Here's the drawing with two shaded views (mm, measured from the low corner). I have some questions. Coordinates: 2 decimals unless noted, no trailing zeros. Loops run counter-clockwise (first coordinate to the right, second up) from the corner with the lowest first, then second, coordinate; pieces in that order, holes last. Notation, with made-up numbers: (67.5, -38.5) - (109.5, -38.5) arc R20 ccw to (109.5, -26.5) - close; hole circle Ø6 at (66.5, 47.5). An arc over 180 degrees is marked (long way). Use a Markdown table: item, result.
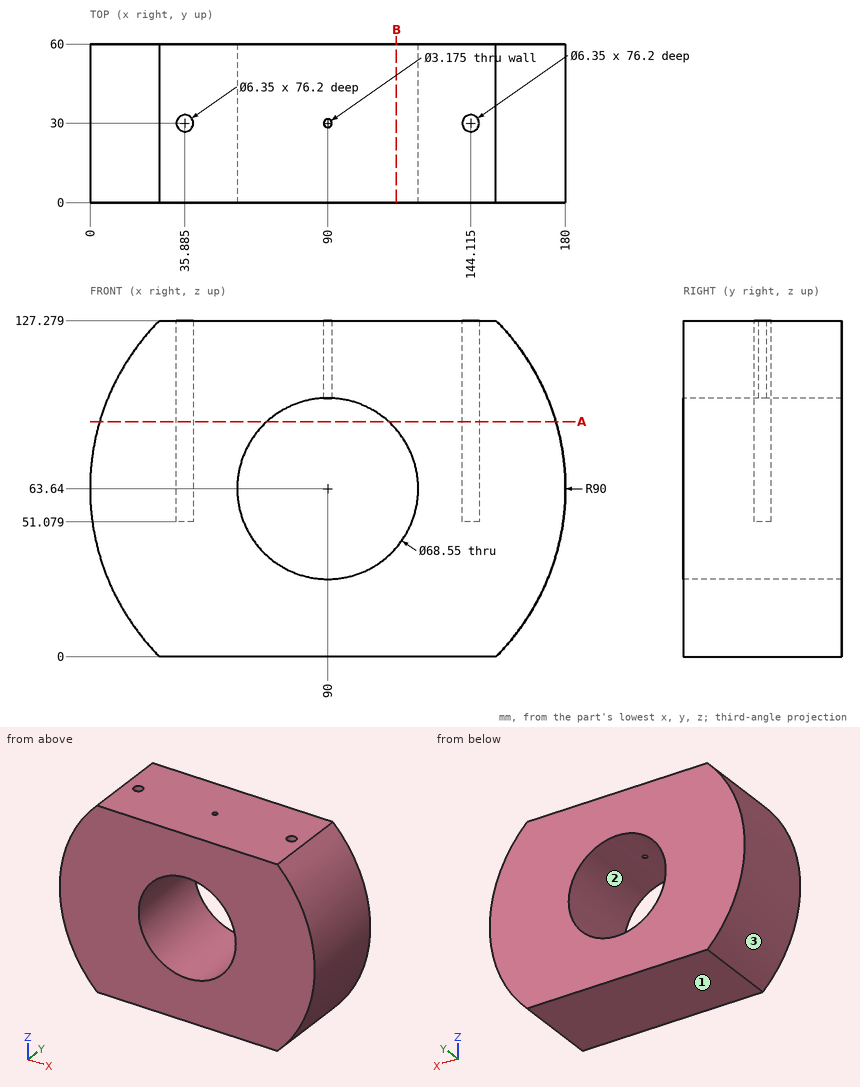
Q1. Please list where these lines run through material, in increasing order: L1, parallel to Y at x = 90, z = 112.5; L2, parallel to X at y = 48, z = 58.5; L3, parallel to Z at x = 62.5, y = 29.5 (1 decimal). Write a range as from..to.
Check values:
| item | result |
|---|---|
| L1 | 0..28.41, 31.59..60 |
| L2 | 0.15..56.11, 123.89..179.85 |
| L3 | 0..43.2, 84.1..127.3 |
Q2. Will these pins go through, and if not, where does the flat tip stop? P1, Ø8.5, axis at x = 35.89, y = 30, coming from the +Z side; P2, Ø1, axis at y = 44, z = 89, coming from the -X side; P3, Ø4, axis at y = 7.5, z = 68, coming from the -X side; P4, Ø2.5, axis at x = 90, y = 30, coming from the +Z side.
Check values:
| item | result |
|---|---|
| P1 | z = 127.28 |
| P2 | x = 3.5 |
| P3 | x = 0.03 |
| P4 | z = 29.39 |
Q3. If we mould it in two halves opening along Z, with no side actions, what happens to the marked faces 1, 2 and 3? For each: pulls with the +Z half, pulls with the -Z half, needs draft (parallel to the pull), parting line crosses it, or undercut.
Check values:
| item | result |
|---|---|
| face 1 | pulls with the -Z half |
| face 2 | undercut |
| face 3 | parting line crosses it |
Q4. I want a section at B-B, the plane x = 116. Write out the boundary of the cut face in (y, z), then the cut area to 3 significant figures.
Check values:
| item | result |
|---|---|
| outline | (0, 0) - (60, 0) - (60, 41.31) - (0, 41.31) - close; (0, 85.97) - (60, 85.97) - (60, 127.28) - (0, 127.28) - close |
| area | 4,960 mm^2 |
Q5. I want a section at A-A, the plane z = 89. Give the number of separate pieces and of enclosed holes in the cut face, then the cut area to 3 significant figures.
Check values:
| item | result |
|---|---|
| separate pieces | 2 |
| enclosed holes | 2 |
| area | 7,530 mm^2 |
